The listing builds one solid part. Answer for the finished solid, in the listing's coordinates (mm). Face numbers are marked on the shaded views. A direction names the side the tool comes from. Round coordinates to 2 decimals unless told otherwise and drop trailing zeros. Write each loop counter-clockwise with the first axis right and the second up, starting at its lowest first coordinate (ties: lowest second). Pieces come first, ordered by that corner, then holes. Notation, with made-up numbers: M 82.25,-21.5 L 123.25,-21.5 A25 ccw 123.25,-0.5 Z; hole C 69,46 d1. An arc over 180 degrees is marked long. One line per item, written item: value. Start each with the question number.
(1) Given P1, Ø6, axis at y = 29.5, z = 11, coming from the +X side, flat-ended and moving along its own axis, determine where the tip first touches the part or whether it passes through.
(2) Section B-B (z = 30.5) is taken. Determine the outline of the cut face in (x, y), plus the area to 3 significant figures.
(3) Section A-A (y = 22.5) is taken. Determine the outline of the cut face in (x, z), plus the area to 3 significant figures.
(4) Section D-D (y = 38.5) is taken. Determine the outline of the cut face in (x, z).
(5) Consider probe 1 along X at (y, z) = (47, 15.5); probe 2 along Z at (x, y) = (121, 50.5); probe 3 along X at (y, z) = (68, 30). Determine where each line is inside the solid, lowest interval first.
(6) For a pull along X with two mould halves and no side action, classify the marked faces 3, 4 and 5 as released by +X, released by -X, zero draft, split by the parting line, or undercut.
(7) Section C-C (y = 64) is taken. Determine the outline of the cut face in (x, z), plus the area to 3 significant figures.
(8) For the marked faces 1 and 2, determine the directions among +Z, -Z, +X, -X, +Y, -Y from which every point of the face is accessible in a straight line to the end or side of a thin tool.
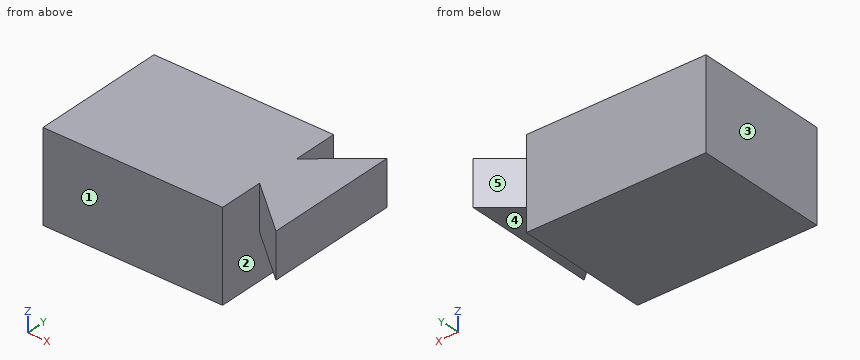
```python
from build123d import *

# Parameters (mm, degrees)
F0_W     = 101.6
F0_H     = 76.2
F1_DEPTH = 50.8
F3_DEPTH = 25.4


with BuildPart() as f1:
    # F0 (on Top) → F1 (new body)
    with BuildSketch(Plane.XY):
        with Locations((50.8, 38.1)):
            Rectangle(F0_W, F0_H)
    extrude(amount=F1_DEPTH)

    # F2 (on face) → F3 (join)
    with BuildSketch(Plane.XY.offset(50.8)):
        Polygon((101.6, 50.8), (101.6, 25.4), (131.798387, 0), (131.798387, 76.2), align=None)
    extrude(amount=-F3_DEPTH)


solid = f1.part
```
Recorded:
1. P1: stops at x = 101.6
2. outline: M 0,0 L 101.6,0 L 101.6,25.4 L 131.8,0 L 131.8,76.2 L 101.6,50.8 L 101.6,76.2 L 0,76.2 Z
2. area: 9,280 mm2
3. outline: M 0,0 L 101.6,0 L 101.6,50.8 L 0,50.8 Z; M 105.05,25.4 L 131.8,25.4 L 131.8,50.8 L 105.05,50.8 Z
3. area: 5,840 mm2
4. outline: M 0,0 L 101.6,0 L 101.6,25.4 L 131.8,25.4 L 131.8,50.8 L 0,50.8 Z
5. probe 1: x = 0 to 101.6
5. probe 2: z = 25.4 to 50.8
5. probe 3: x = 0 to 101.6, 122.05 to 131.8
6. face 3: released by -X
6. face 4: zero draft
6. face 5: undercut
7. outline: M 0,0 L 101.6,0 L 101.6,50.8 L 0,50.8 Z; M 117.29,25.4 L 131.8,25.4 L 131.8,50.8 L 117.29,50.8 Z
7. area: 5,530 mm2
8. face 1: +Z, -Z, +X, -X, -Y
8. face 2: -Z
